```python
from build123d import *

# Parameters (mm, degrees)
SALIENTE_EXTRUIR1_DEPTH = 250


with BuildPart() as part:
    # Croquis1 → Saliente-Extruir1 (new, symmetric)
    with BuildSketch(Plane.XY):
        with BuildLine():
            Line((0, 2), (0, 40))
            Line((0, 40), (-4, 40))
            Line((-4, 40), (-4, -4))
            Line((-4, -4), (40, -4))
            Line((40, -4), (40, 0))
            Line((40, 0), (2, 0))
            ThreePointArc((2, 0), (0.585786438, 0.585786438), (0, 2))
        make_face()
    extrude(amount=SALIENTE_EXTRUIR1_DEPTH, both=True)


solid = part.part
```
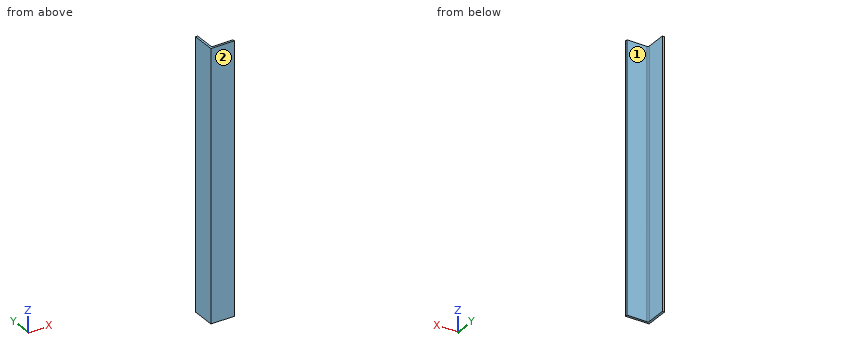
Geometry: final body of the model. Coordinates: model frame, mm. Face numbers are marked on the shaded views. A direction names the side the tool comes from. Coordinates: 2 decimals unless noted, no trailing zeros. Order: outer loops, then holes, each group sorted by start corner. A loop starts at its lowest first (then second) coordinate and runs counter-clockwise, first axis right, second up.
Item 1: Contact query for flat-ended pins moving along their axis: P1, Ø6, axis at y = 15, z = -141, coming from the +X side; P2, Ø11.5, axis at x = 20.5, z = 20.5, coming from the +Y side. Output: stop coordinate, or through.
Answer:
P1: stops at x = 0
P2: stops at y = 0
Item 2: Material intervals for line 1 along X through (y, z) = (32.5, -171.5); line 2 along Y through (x, z) = (1.5, 134), sorted ascending.
Answer:
line 1: x = -4 to 0
line 2: y = -4 to 0.06
Item 3: Access query for the marked faces 1 and 2. Directions: +Z, -Z, +X, -X, +Y, -Y. A direction counts if a zero-diameter tool reaches every point of the face in a straight line with its end or side. Return the directions, or none.
Answer:
face 1: +Z, -Z, +X, +Y
face 2: +Z, -Z, +X, -X, -Y
Item 4: Section query B-B (y = 7.5). Output: boundary loops of the cut face in (x, z).
Answer:
outline: (-4, -250) - (0, -250) - (0, 250) - (-4, 250) - close
Item 5: Section query A-A (z = 121). Output: boundary loops of the cut face in (x, y).
Answer:
outline: (-4, -4) - (40, -4) - (40, 0) - (2, 0) arc R2 cw to (0, 2) - (0, 40) - (-4, 40) - close
